from build123d import *

# Parameters (mm, degrees)
SKETCH1_W           = 22
SKETCH1_H           = 3
BOSS_EXTRUDE1_DEPTH = 13.9
SKETCH1_3_W         = 6.1
SKETCH1_3_H         = 32.8
BOSS_EXTRUDE2_DEPTH = 20
SKETCH2_R           = 2
CUT_EXTRUDE1_DEPTH  = 42.7708032


with BuildPart() as part:
    # Sketch1 → Boss-Extrude1 (new body)
    with BuildSketch(Plane.XY):
        Polygon((-16.4, -8), (-16.4, -16.4), (10.3, -16.4), (10.3, 16.4), (-16.4, 16.4), (-16.4, 8), (7.6, 8), (7.6, -8), align=None)
        with Locations((-3.4, -12.4)):
            Rectangle(SKETCH1_W, SKETCH1_H, mode=Mode.SUBTRACT)
        with Locations((-3.4, 12.4)):
            Rectangle(SKETCH1_W, SKETCH1_H, mode=Mode.SUBTRACT)
    extrude(amount=BOSS_EXTRUDE1_DEPTH)

    # Sketch1<3> → Boss-Extrude2 (add)
    with BuildSketch(Plane.XY):
        with Locations((13.35, 0)):
            Rectangle(SKETCH1_3_W, SKETCH1_3_H)
    extrude(amount=BOSS_EXTRUDE2_DEPTH)

    # Sketch2 → Cut-Extrude1 (cut, through all)
    with BuildSketch(Plane(origin=(16.4, 0, 0), x_dir=(0, 0, -1), z_dir=(1, 0, 0))):
        with Locations((-6.95, 8.2)):
            Circle(SKETCH2_R)
        with Locations((-6.95, -8.2)):
            Circle(SKETCH2_R)
    extrude(amount=-CUT_EXTRUDE1_DEPTH, mode=Mode.SUBTRACT)


solid = part.part
The listing builds one solid part. Answer for the finished solid, in the listing's coordinates (mm). A direction names the side the tool comes from. Round coordinates to 2 decimals unless told otherwise and drop trailing zeros. Write each loop counter-clockwise with the first axis right and the second up, starting at its lowest first coordinate (ties: lowest second). Pieces come first, ordered by that corner, then holes. Notation, with made-up numbers: M 2.25,-5.75 L 27.25,-5.75 A11 ccw 27.25,9.25 Z; hole C -6,89 d7. An arc over 180 degrees is marked long. Write each question's results on one line, items separated by ' | '. Start each with the question number.
Item 1: Given pin 1 Ø4 at (y, z) = (3.5, 11) entering from -X; pin 2 Ø1 at (x, y) = (9.5, 10.5) entering from +Z, each flat-ended and moving along its own axis, determine where each tip first touches the part or whether it passes through.
Item 2: Which of the six approach directions +Z, -Z, +X, -X, +Y, -Y give full straight-line access (tool end or side, diameter ignored) to faces 1 (the flat face through (-4, 10.9, 7)), 2 (the flat face through (0, -16.4, 8)), 3 (the flat face through (-5, 8, 2))?
Item 3: The mould has two halves that part along Z. Classify faces 4 (the flat face through (-14.4, 12, 7)), 5 (the flat face through (-0.3, -10.7, 13.9)), 6 (the cylindrical face through (3.874, -10.152, 7.384)): +Z half, -Z half, draft (parallel to the pull), parting line (faces both ways), or undercut.
Item 4: Find section D-D on y = 12. Write down the section's boundary in (x, z).
Item 5: Find section B-B on z = 6.95. Write down the section's boundary in (x, y).
Item 6: Straight lines are drawn through the part: probe 1 along Y at (x, z) = (3, 6.95); probe 2 along Y at (x, z) = (-9, 1.5); probe 3 along X at (y, z) = (-12, 9.25). For each, find the intervals that lie inside material, in ascending order.
Item 7: Find section A-A on y = 7. Write down the section's boundary in (x, z), and give its area (3 significant figures).
Item 8: Find section C-C on x = -2.5. Write down the section's boundary in (y, z).
Answer block:
1) pin 1: stops at x = 7.6 | pin 2: stops at z = 13.9
2) face 1: +Z, -Z | face 2: +Z, -Z, +X, -X, -Y | face 3: +Z, -Z, -X
3) face 4: draft | face 5: +Z half | face 6: undercut
4) outline: M -16.4,0 L -14.4,0 L -14.4,13.9 L -16.4,13.9 Z; M 7.6,0 L 16.4,0 L 16.4,20 L 10.3,20 L 10.3,13.9 L 7.6,13.9 Z
5) outline: M -16.4,-16.4 L 16.4,-16.4 L 16.4,-10.2 L -16.4,-10.2 Z; M -16.4,10.2 L 16.4,10.2 L 16.4,16.4 L -16.4,16.4 Z; M 7.6,-6.2 L 16.4,-6.2 L 16.4,6.2 L 7.6,6.2 Z; hole M -14.4,-13.9 L 7.6,-13.9 L 7.6,-10.9 L -14.4,-10.9 Z; hole M -14.4,10.9 L 7.6,10.9 L 7.6,13.9 L -14.4,13.9 Z
6) probe 1: y = -16.4 to -13.9, -10.9 to -10.2, 10.2 to 10.9, 13.9 to 16.4 | probe 2: y = -16.4 to -13.9, -10.9 to -8, 8 to 10.9, 13.9 to 16.4 | probe 3: x = -16.4 to -14.4, 7.6 to 16.4
7) outline: M 7.6,0 L 16.4,0 L 16.4,5.35 L 7.6,5.35 Z; M 7.6,8.55 L 16.4,8.55 L 16.4,20 L 10.3,20 L 10.3,13.9 L 7.6,13.9 Z | area: 131 mm²
8) outline: M -16.4,0 L -13.9,0 L -13.9,13.9 L -16.4,13.9 Z; M -10.9,0 L -8,0 L -8,4.96 A2 cw long -8,8.94 L -8,13.9 L -10.9,13.9 Z; M 8,0 L 10.9,0 L 10.9,13.9 L 8,13.9 L 8,8.94 A2 cw long 8,4.96 Z; M 13.9,0 L 16.4,0 L 16.4,13.9 L 13.9,13.9 Z
